Geometry: see drawing. Coordinates: mm, zero at the bounding-box minimum. Coordinates: 2 decimals unless noted, no trailing zeros. Write each loop counter-clockwise with the first axis right and the second up, starting at its lowest first coordinate (ties: lowest second). Pieces come first, ordered by that corner, then holes. Notation, with made-up numbers: M -31.5,76.25 L -13.5,76.25 A33 ccw -13.5,108.25 Z; hole C 44,-28 d9. An arc over 180 degrees is marked long. One line per item, written item: value. Start each with the question number.
Item 1: Pin query (flat end, axial travel): P1, Ø1.2, axis at x = 23.52, z = 44.45, coming from the +Y side; P2, Ø10.5, axis at x = 15, z = 12.5, coming from the +Y side. Return the tip coordinate at first contact, or that it passes through.
Item 2: Cut plane C-C, the plane x = 31. Output: boundary loops of the cut face in (y, z).
Item 3: Cut plane B-B, the plane y = 0.8. Output: boundary loops of the cut face in (x, z), then the cut area to 3 significant figures.
Item 4: Cut plane D-D, the plane x = 6.3. Output: boundary loops of the cut face in (y, z).
Item 5: Ray query, L1, parallel to X at y = 0.9, z = 3.81; L2, parallel to Z at x = 30.48, y = 0.6; L3, parallel to X at y = 0.85, z = 44.45. Return the intervals inside material, ascending. Write a range as from..to.
Item 6: Cut plane A-A, the plane x = 10.77. Output: boundary loops of the cut face in (y, z), then the cut area to 3 significant figures.
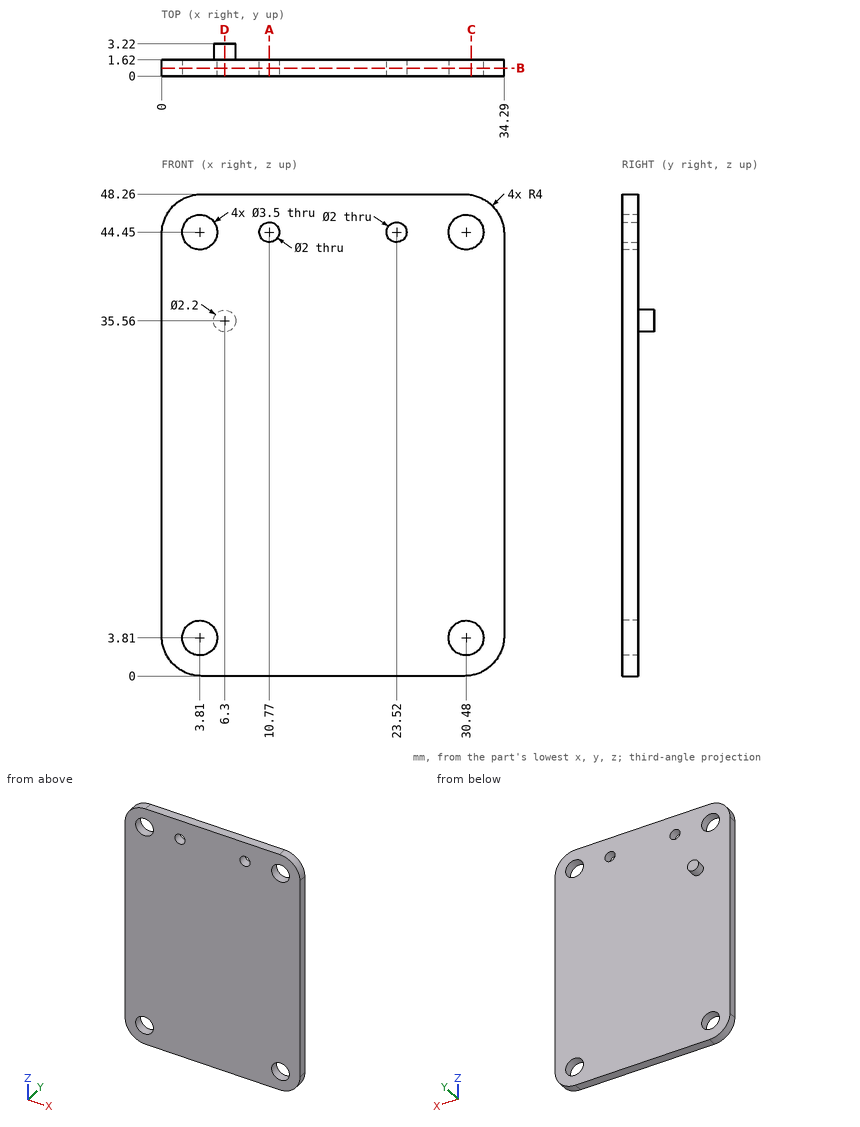
From the geometry:
1. P1: passes through
1. P2: stops at y = 1.62
2. outline: M 0,0.06 L 1.62,0.06 L 1.62,2.14 L 0,2.14 Z; M 0,5.48 L 1.62,5.48 L 1.62,42.78 L 0,42.78 Z; M 0,46.12 L 1.62,46.12 L 1.62,48.2 L 0,48.2 Z
3. outline: M 0,4 A4 ccw 4,0 L 30.29,0 A4 ccw 34.29,4 L 34.29,44.26 A4 ccw 30.29,48.26 L 4,48.26 A4 ccw 0,44.26 Z; hole C 3.81,3.81 d3.5; hole C 3.81,44.45 d3.5; hole C 10.77,44.45 d2; hole C 23.52,44.45 d2; hole C 30.48,3.81 d3.5; hole C 30.48,44.45 d3.5
3. area: 1,600 mm²
4. outline: M 0,0 L 1.62,0 L 1.62,34.46 L 3.22,34.46 L 3.22,36.66 L 1.62,36.66 L 1.62,48.26 L 0,48.26 Z
5. L1: x = 0..2.06, 5.56..28.73, 32.23..34.29
5. L2: z = 0..2.06, 5.56..42.7, 46.2..48.26
5. L3: x = 0..2.06, 5.56..9.77, 11.77..22.52, 24.52..28.73, 32.23..34.29
6. outline: M 0,0 L 1.62,0 L 1.62,43.45 L 0,43.45 Z; M 0,45.45 L 1.62,45.45 L 1.62,48.26 L 0,48.26 Z
6. area: 74.9 mm²
